For this review, take the finished solid that the model builds, in its own axes (mm). A direction names the side the tool comes from. Coordinates: 2 decimals unless noted, no trailing zeros. Loops run counter-clockwise (first coordinate to the right, second up) from the corner with the lowest first, then second, coordinate; pieces in that order, holes last. Notation, with made-up numbers: M -25.5,72.5 L 2.5,72.5 A17 cw 2.5,97.5 Z; hole C 16.25,28.25 d5. An arc over 180 degrees is marked long. Put each result on its own line as item: value.
```python
from build123d import *

# Parameters (mm, degrees)
SKETCH_1_R      = 1.5
EXTRUDE_1_DEPTH = 1
CHAMFER_1_SIZE  = 10


with BuildPart() as part:
    # 草图1 → 凸台-拉伸1 (new body)
    with BuildSketch(Plane.XY):
        Polygon((0, 0), (0, 110), (240, 110), (240, 0), (227.5, 0), (227.5, 90), (82.5, 90), (82.5, 0), align=None)
        with Locations((10, 107)):
            Circle(SKETCH_1_R, mode=Mode.SUBTRACT)
        with Locations((30, 107)):
            Circle(SKETCH_1_R, mode=Mode.SUBTRACT)
        with Locations((210, 107)):
            Circle(SKETCH_1_R, mode=Mode.SUBTRACT)
        with Locations((230, 107)):
            Circle(SKETCH_1_R, mode=Mode.SUBTRACT)
        with Locations(Location((80, 107, 0), (0, 0, 180))):
            Circle(SKETCH_1_R, mode=Mode.SUBTRACT)
        with Locations(Location((100, 107, 0), (0, 0, 180))):
            Circle(SKETCH_1_R, mode=Mode.SUBTRACT)
    extrude(amount=EXTRUDE_1_DEPTH)

    # 倒角1
    chamfer_1_edges = [part.edges().sort_by_distance(p)[0] for p in [
        (227.5, 90, 0.5),
        (82.5, 90, 0.5),
    ]]
    chamfer(chamfer_1_edges, length=CHAMFER_1_SIZE)


solid = part.part
```
(1) Add section B-B (z = 0.5). Write out the cut boundary in (x, y), plus the area to 3 significant figures.
Determined:
outline: M 0,0 L 82.5,0 L 82.5,80 L 92.5,90 L 217.5,90 L 227.5,80 L 227.5,0 L 240,0 L 240,110 L 0,110 Z; hole C 10,107 d3; hole C 30,107 d3; hole C 80,107 d3; hole C 100,107 d3; hole C 210,107 d3; hole C 230,107 d3
area: 13,400 mm^2
(2) Wall thickness on line 1 along Y through (x, z) = (230, 0.35); line 2 along X through (y, z) = (46, 0.85); line 3 along Y through (x, z) = (210, 0.85): over which ranges is each line inside the solid? List them lowest first. Write a range as [from, to].
Determined:
line 1: y = [0, 105.5], [108.5, 110]
line 2: x = [0, 82.5], [227.5, 240]
line 3: y = [90, 105.5], [108.5, 110]
(3) Draft analysis for pull direction X (two halves, no side actions). For faces 1 (the flat face through (95, 92, 1)), 2 (the flat face through (87.6, 85.1, 0.5)), state which applies: +X half, -X half, draft (parallel to the pull), parting line (faces both ways), or undercut.
Determined:
face 1: draft
face 2: undercut
(4) Add section C-C (y = 84). Write out the cut boundary in (x, z).
Determined:
outline: M 0,0 L 86.5,0 L 86.5,1 L 0,1 Z; M 223.5,0 L 240,0 L 240,1 L 223.5,1 Z
(5) Tool access review of faces 3 (the flat face through (222.6, 84.9, 0.5)), 4 (the flat face through (95, 92, 0)): name each direction out of +Z, -Z, +X, -X, +Y, -Y from which nothing blocks a thin tool from reaching the whole face with its end or side.
Determined:
face 3: +Z, -Z, -Y
face 4: -Z, +X, -X, +Y, -Y
(6) Add section A-A (y = 40.5). Write out the cut boundary in (x, z), plus the area to 3 significant figures.
Determined:
outline: M 0,0 L 82.5,0 L 82.5,1 L 0,1 Z; M 227.5,0 L 240,0 L 240,1 L 227.5,1 Z
area: 95.0 mm^2
(7) Add section D-D (x = 88). Write out the cut boundary in (y, z), plus the area to 3 significant figures.
Determined:
outline: M 85.5,0 L 110,0 L 110,1 L 85.5,1 Z
area: 24.5 mm^2
